Geometry check sheet. Reference: the model listing, model coordinates, mm. A direction names the side the tool comes from. Give positions to 0.01 mm unless a question says otherwise; leave off trailing zeros. Loops run counter-clockwise (first coordinate to the right, second up) from the corner with the lowest first, then second, coordinate; pieces in that order, holes last. Notation, with made-up numbers: (-34.75, 74.25) - (-28.75, 74.25) arc R30 ccw to (-28.75, 99.25) - close; hole circle Ø2 at (88, -6.5). An arc over 180 degrees is marked (long way). Use a Markdown table: item, result. Add a question column.
1. Cross-section at C-C on x = 8.75. Enter the section's corners in (y, z).
2. Cross-section at B-B on z = -26.7. Enter the section's corners in (x, y), and give its area (3 significant figures).
3. Cross-section at A-A on y = 3. Enter the section's corners in (x, z).
4. Depth check by flat-ended pin: P1, Ø2, axis at x = 8, z = 2.5, coming from the -Y side; P2, Ø1.5, axis at x = 6.5, z = 6, coming from the -Y side; P3, Ø1.9, axis at y = 3, z = 4, coming from the +X side; P4, Ø2, axis at y = 1.5, z = -2.5, coming from the -X side. Enter the tip coordinate at first touch or a pass-through.
5. Set-up check for faces 1 (the flat face through (6, 0, 6)), 2 (the cylindrical face through (7.1, -1.25, -27.07)), 3 (the flat face through (0.55, 4.43, 3.7)), 4 (the flat face through (0.75, 2, -24)), 5 (the flat face through (6, 3, 0)): record each of +Z, -Z, +X, -X, +Y, -Y from which the full face is reachable in a straight line by a thin tool's end or side.
6. Draft check along X on faces 6 (the flat face through (0, 2, 4)), 7 (the flat face through (6, 5, 4)), 8 (the flat face through (11.7, 2, 4)), 9 (the cylindrical face through (4.6, -1.25, -27.07)). Enter one of: pulls with the +X half, pulls with the -X half, needs draft (parallel to the pull), parting line crosses it, or undercut.
7. Cross-section at D-D on z = 3.5. Enter the section's corners in (x, y), and give its area (3 significant figures).
8. Material ranges on L1, parallel to Z at x = 10.5, y = 3.25; L2, parallel to Z at x = 2, y = -1; L3, parallel to Y at x = 10, z = -19.5, recorded low to high.
from build123d import *

# Parameters (mm, degrees)
DODANIE_WYCI_GNI_CIE1_DEPTH = 7.5
SZKIC2_W                    = 13
SZKIC2_H                    = 34
DODANIE_WYCI_GNI_CIE2_DEPTH = 0.41
SZKIC3_R                    = 0.3
DODANIE_WYCI_GNI_CIE3_DEPTH = 1.69
SZKIC4_W                    = 10.5
SZKIC4_H                    = 10
DODANIE_WYCI_GNI_CIE4_DEPTH = 5
SZKIC6_R                    = 0.4
DODANIE_WYCI_GNI_CIE5_DEPTH = 1.7


with BuildPart() as part:
    # Szkic1 → Dodanie-wyciągnięcie1 (new body)
    with BuildSketch(Plane.XY):
        Polygon((10.58, 5), (11.7, 3.88), (11.7, 0), (0, 0), (0, 3.88), (1.12, 5), align=None)
    extrude(amount=DODANIE_WYCI_GNI_CIE1_DEPTH)

    # Szkic2 → Dodanie-wyciągnięcie2 (add)
    with BuildSketch(Plane.XZ):
        with Locations((6, -12.45)):
            Rectangle(SZKIC2_W, SZKIC2_H)
    extrude(amount=DODANIE_WYCI_GNI_CIE2_DEPTH)

    # Szkic3 → Dodanie-wyciągnięcie3 (add)
    with BuildSketch(Plane.XZ.offset(0.41)):
        with Locations(Location((2.255290514, 0.3, 0), (0, 0, 270))):
            Circle(SZKIC3_R)
        with Locations(Location((4.755290514, 0.3, 0), (0, 0, 270))):
            Circle(SZKIC3_R)
        with Locations(Location((7.255290514, 0.3, 0), (0, 0, 270))):
            Circle(SZKIC3_R)
        with Locations(Location((9.755290514, 0.3, 0), (0, 0, 270))):
            Circle(SZKIC3_R)
    extrude(amount=DODANIE_WYCI_GNI_CIE3_DEPTH)

    # Szkic4 → Dodanie-wyciągnięcie4 (add)
    with BuildSketch(Plane(origin=(0, 0, 0), x_dir=(1, 0, 0), z_dir=(0, 1, 0))):
        with Locations((6, 24.55)):
            Rectangle(SZKIC4_W, SZKIC4_H)
    extrude(amount=DODANIE_WYCI_GNI_CIE4_DEPTH)

    # Szkic6 → Dodanie-wyciągnięcie5 (add)
    with BuildSketch(Plane.XZ.offset(0.41)):
        with Locations(Location((2.255290514, -26.7, 0), (0, 0, 270))):
            Circle(SZKIC6_R)
        with Locations(Location((4.755290514, -26.7, 0), (0, 0, 270))):
            Circle(SZKIC6_R)
        with Locations(Location((7.255290514, -26.7, 0), (0, 0, 270))):
            Circle(SZKIC6_R)
        with Locations(Location((9.755290514, -26.7, 0), (0, 0, 270))):
            Circle(SZKIC6_R)
        with Locations(Location((4.755290514, -21.7, 0), (0, 0, 270))):
            Circle(SZKIC6_R)
        with Locations(Location((7.255290514, -21.7, 0), (0, 0, 270))):
            Circle(SZKIC6_R)
        with Locations(Location((9.755290514, -21.7, 0), (0, 0, 270))):
            Circle(SZKIC6_R)
        with Locations(Location((2.255290514, -21.7, 0), (0, 0, 270))):
            Circle(SZKIC6_R)
    extrude(amount=DODANIE_WYCI_GNI_CIE5_DEPTH)


solid = part.part
Values found:
| question | item | result |
|---|---|---|
| 1 | outline | (-0.41, -29.45) - (0, -29.45) - (0, -29.55) - (5, -29.55) - (5, -19.55) - (0, -19.55) - (0, 0) - (5, 0) - (5, 7.5) - (0, 7.5) - (0, 4.55) - (-0.41, 4.55) - close |
| 2 | outline | (-0.5, -0.41) - (1.86, -0.41) - (1.86, -2.11) - (2.66, -2.11) - (2.66, -0.41) - (4.36, -0.41) - (4.36, -2.11) - (5.16, -2.11) - (5.16, -0.41) - (6.86, -0.41) - (6.86, -2.11) - (7.66, -2.11) - (7.66, -0.41) - (9.36, -0.41) - (9.36, -2.11) - (10.16, -2.11) - (10.16, -0.41) - (12.5, -0.41) - (12.5, 0) - (11.25, 0) - (11.25, 5) - (0.75, 5) - (0.75, 0) - (-0.5, 0) - close |
| 2 | area | 63.3 mm2 |
| 3 | outline | (0, 0) - (11.7, 0) - (11.7, 7.5) - (0, 7.5) - close; (0.75, -29.55) - (11.25, -29.55) - (11.25, -19.55) - (0.75, -19.55) - close |
| 4 | P1 | stops at y = -0.41 |
| 4 | P2 | stops at y = 0 |
| 4 | P3 | stops at x = 11.7 |
| 4 | P4 | passes through |
| 5 | face 1 | +Z, +X, -X, -Y |
| 5 | face 2 | -Y |
| 5 | face 3 | +Z, -X, +Y |
| 5 | face 4 | -Z, -X, +Y |
| 5 | face 5 | +X, -X, +Y |
| 6 | face 6 | pulls with the -X half |
| 6 | face 7 | needs draft |
| 6 | face 8 | pulls with the +X half |
| 6 | face 9 | undercut |
| 7 | outline | (-0.5, -0.41) - (12.5, -0.41) - (12.5, 0) - (11.7, 0) - (11.7, 3.88) - (10.58, 5) - (1.12, 5) - (0, 3.88) - (0, 0) - (-0.5, 0) - close |
| 7 | area | 62.6 mm2 |
| 8 | L1 | z = -29.55 to -19.55, 0 to 7.5 |
| 8 | L2 | z = -27.01 to -26.39, -22.01 to -21.39, 0.14 to 0.46 |
| 8 | L3 | y = -0.41 to 0 |
